Part model, mm, in its own coordinate system. Face numbers are marked on the shaded views. A direction names the side the tool comes from. Round coordinates to 2 decimals unless told otherwise and drop trailing zeros. Loops run counter-clockwise (first coordinate to the right, second up) from the corner with the lowest first, then second, coordinate; pieces in that order, holes last.
(1) Tool access for the marked faces 1 and 2: list every direction of +Z, -Z, +X, -X, +Y, -Y with a clear straight run to the whole face (end or side of a thin tool).
(2) Cut at A-A on x = 0. List the corners of the cut face in (y, z), then the cut area to 3 significant figures.
(3) Cut at D-D on x = -4.5. List the corners of the cut face in (y, z).
(4) Flat gauge pins, fed straight in: pin 1 (1.3 mm diameter, centred on y = -5, z = 2, fed in from +X); pin 2 (6.5 mm diameter, centred on x = 2, z = 10, fed in from -Y); pin 3 (3.5 mm diameter, centred on y = -6, z = 3, fed in from +X). Where does each tip first touch, or does it go through?
(5) Cut at B-B on x = 6.5. List the corners of the cut face in (y, z).
(6) Probe probe 1 along X at (y, z) = (-4.5, 1.2); probe 2 along X at (y, z) = (12.8, 9); probe 3 along Y at (x, z) = (-7, 2). List the from-to ranges inside material, lowest first.
(7) Cut at C-C on y = -4.5. Count the separate pieces of the cut face and the enclosed holes in it, then the cut area to 3 significant figures.
(8) Mould opens along Y. For the marked faces 3, 4, 5 and 6 say: +Y half, -Y half, draft (parallel to the pull), parting line (faces both ways), or undercut.
from build123d import *

# Parameters (mm, degrees)
SKETCH1_W                               = 18
SKETCH1_H                               = 30
BOSS_EXTRUDE1_DEPTH                     = 3
SKETCH3_W                               = 18
SKETCH3_H                               = 3
BOSS_EXTRUDE2_DEPTH                     = 9
CBORE_FOR_M5_HEX_HEAD_BOLT1_D           = 4
CBORE_FOR_M5_HEX_HEAD_BOLT1_DEPTH       = 4
CBORE_FOR_M5_HEX_HEAD_BOLT1_CBORE_D     = 5
CBORE_FOR_M5_HEX_HEAD_BOLT1_CBORE_DEPTH = 0.8
CBORE_FOR_M5_HEX_HEAD_BOLT1_TIP         = 1.178090033
CHAMFER1_SIZE                           = 1
SKETCH8_W                               = 18
SKETCH8_H                               = 6
CUT_EXTRUDE1_DEPTH                      = 12
FILLET2_R                               = 0.5
F_3_0MM_DOWEL_HOLE1_D                   = 3
F_3_0MM_DOWEL_HOLE1_DEPTH               = 10
F_3_0MM_DOWEL_HOLE1_TIP                 = 0.901290929


with BuildPart() as part:
    # Sketch1 → Boss-Extrude1 (new body)
    with BuildSketch(Plane.XY):
        Rectangle(SKETCH1_W, SKETCH1_H)
    extrude(amount=BOSS_EXTRUDE1_DEPTH)

    # Sketch2 → Cut-Revolve1 (revolve, cut)
    with BuildSketch(Plane.XY.offset(3)):
        Polygon((6.8, 8.5), (6, 8.5), (6, 6), (9, 6), (9, 8.5), (8.2, 8.5), (8.2, 8), (6.8, 8), align=None)
    cut_revolve1 = revolve(axis=Axis((6.04728637, 6, 3), (1, 0, 0)), mode=Mode.SUBTRACT)

    # Sketch2<3> → Revolve1 (revolve)
    with BuildSketch(Plane.XY.offset(3), mode=Mode.PRIVATE) as revolve1_sk:
        Polygon((6.8, 9), (6.8, 8.5), (6.8, 8), (8.2, 8), (8.2, 8.5), (9, 8.5), (9, 9), align=None)
    revolve1 = revolve(revolve1_sk.sketch.rotate(Axis((6.04728637, 6, 3), (1, 0, 0)), 90), axis=Axis((6.04728637, 6, 3), (1, 0, 0)))

    # Mirror1: Cut-Revolve1, Revolve1 across plane
    add(cut_revolve1.mirror(Plane(origin=(0, 0, 0), x_dir=(0, 0, 1), z_dir=(1, 0, 0))), mode=Mode.SUBTRACT)
    add(revolve1.mirror(Plane(origin=(0, 0, 0), x_dir=(0, 0, 1), z_dir=(1, 0, 0))))

    # Mirror2: Cut-Revolve1, Revolve1 across plane
    add(cut_revolve1.mirror(Plane.ZX), mode=Mode.SUBTRACT)
    add(revolve1.mirror(Plane.ZX))

    # Mirror2 copy 1 sketch → Mirror2 copy 1 (revolve, cut)
    with BuildSketch(Plane(origin=(0, 0, 3), x_dir=(-1, 0, 0), z_dir=(0, 0, 1))):
        Polygon((6.8, 8.5), (6, 8.5), (6, 6), (9, 6), (9, 8.5), (8.2, 8.5), (8.2, 8), (6.8, 8), align=None)
    revolve(axis=Axis((-6.04728637, -6, 3), (-1, 0, 0)), mode=Mode.SUBTRACT)

    # Mirror2 copy 2 sketch → Mirror2 copy 2 (revolve)
    with BuildSketch(Plane(origin=(0, 0, 3), x_dir=(-1, 0, 0), z_dir=(0, 0, 1))):
        Polygon((6.8, 9), (6.8, 8.5), (6.8, 8), (8.2, 8), (8.2, 8.5), (9, 8.5), (9, 9), align=None)
    revolve(axis=Axis((-6.04728637, -6, 3), (-1, 0, 0)))

    # Sketch3 → Boss-Extrude2 (add)
    with BuildSketch(Plane.XY.offset(3)):
        with Locations((0, 13.5)):
            Rectangle(SKETCH3_W, SKETCH3_H)
    extrude(amount=BOSS_EXTRUDE2_DEPTH)

    # CBORE for M5 Hex Head Bolt1
    with Locations(Plane(origin=(0, 15, 0), x_dir=(1, 0, 0), z_dir=(0, 1, 0))):
        with Locations((-6, -9), (6, -9)):
            CounterBoreHole(CBORE_FOR_M5_HEX_HEAD_BOLT1_D / 2, CBORE_FOR_M5_HEX_HEAD_BOLT1_CBORE_D / 2, CBORE_FOR_M5_HEX_HEAD_BOLT1_CBORE_DEPTH, depth=CBORE_FOR_M5_HEX_HEAD_BOLT1_DEPTH)
            with Locations((0, 0, -(CBORE_FOR_M5_HEX_HEAD_BOLT1_DEPTH + CBORE_FOR_M5_HEX_HEAD_BOLT1_TIP / 2))):  # 119° drill point
                Cone(0, CBORE_FOR_M5_HEX_HEAD_BOLT1_D / 2, CBORE_FOR_M5_HEX_HEAD_BOLT1_TIP, mode=Mode.SUBTRACT)

    # Chamfer1
    chamfer1_edges = [part.edges().sort_by_distance(p)[0] for p in [
        (0, 12, 3),
        (0, 15, 0),
    ]]
    chamfer(chamfer1_edges, length=CHAMFER1_SIZE)

    # Sketch8 → Cut-Extrude1 (cut)
    with BuildSketch(Plane(origin=(0, 0, 0), x_dir=(-1, 0, 0), z_dir=(0, 0, -1))):
        with Locations((0, -12)):
            Rectangle(SKETCH8_W, SKETCH8_H)
    extrude(amount=-CUT_EXTRUDE1_DEPTH, mode=Mode.SUBTRACT)

    # Fillet2
    # the kernel refuses this fillet: 0.5 mm, written as the material it takes off along each edge
    with BuildSketch(Plane(origin=(-10.25, 15, 12), x_dir=(0, 0, -1), z_dir=(1, 0, 0))) as fillet2_piece_1:
        with BuildLine():
            CenterArc((FILLET2_R, -FILLET2_R), FILLET2_R, 90, 90)
            Line((0, -FILLET2_R), (0, 0))
            Line((0, 0), (FILLET2_R, 0))
        make_face()
    extrude(amount=20.5, mode=Mode.SUBTRACT)
    with BuildSketch(Plane(origin=(-9, 6.000000014, 0), x_dir=(1, 0, 0), z_dir=(0, -1, 0))) as fillet2_piece_2:
        with BuildLine():
            CenterArc((FILLET2_R, FILLET2_R), FILLET2_R, 180, 90)
            Line((0, FILLET2_R), (0, 0))
            Line((0, 0), (FILLET2_R, 0))
        make_face()
    extrude(amount=12.000000014, mode=Mode.SUBTRACT)
    with BuildSketch(Plane(origin=(-9, 15.883883476, 1.883883476), x_dir=(0, -0.7071067811865476, 0.7071067811865476), z_dir=(0, -0.7071067811865476, -0.7071067811865476)), Plane(origin=(9, 15.883883476, 1.883883476), x_dir=(-1, 0, 0), z_dir=(0, -0.7071067811865476, -0.7071067811865476))) as fillet2_piece_3:
        with BuildLine():
            CenterArc((FILLET2_R, -FILLET2_R), FILLET2_R, 90, 90)
            Line((0, -FILLET2_R), (0, 0))
            Line((0, 0), (FILLET2_R, 0))
        make_face()
    extrude(amount=3.914213562, mode=Mode.SUBTRACT)
    with BuildSketch(Plane(origin=(9, -6.000000014, 0), x_dir=(-1, 0, 0), z_dir=(0, 1, 0))) as fillet2_piece_4:
        with BuildLine():
            CenterArc((FILLET2_R, FILLET2_R), FILLET2_R, 180, 90)
            Line((0, FILLET2_R), (0, 0))
            Line((0, 0), (FILLET2_R, 0))
        make_face()
    extrude(amount=12.000000015, mode=Mode.SUBTRACT)
    with BuildSketch(Plane(origin=(10.25, -9, 0), x_dir=(0, 0, 1), z_dir=(-1, 0, 0))) as fillet2_piece_5:
        with BuildLine():
            CenterArc((FILLET2_R, FILLET2_R), FILLET2_R, 180, 90)
            Line((0, FILLET2_R), (0, 0))
            Line((0, 0), (FILLET2_R, 0))
        make_face()
    extrude(amount=20.5, mode=Mode.SUBTRACT)
    with BuildSketch(Plane(origin=(9, 15, 13.25), x_dir=(-1, 0, 0), z_dir=(0, 0, -1)), Plane(origin=(-9, 15, -0.25), x_dir=(1, 0, 0), z_dir=(0, 0, 1))) as fillet2_piece_6:
        with BuildLine():
            CenterArc((FILLET2_R, -FILLET2_R), FILLET2_R, 90, 90)
            Line((0, -FILLET2_R), (0, 0))
            Line((0, 0), (FILLET2_R, 0))
        make_face()
    extrude(amount=13.5, mode=Mode.SUBTRACT)
    with BuildSketch(Plane(origin=(9, -10.25, 0), x_dir=(-1, 0, 0), z_dir=(0, 1, 0))) as fillet2_piece_7:
        with BuildLine():
            CenterArc((FILLET2_R, FILLET2_R), FILLET2_R, 180, 90)
            Line((0, FILLET2_R), (0, 0))
            Line((0, 0), (FILLET2_R, 0))
        make_face()
    extrude(amount=4.249999986, mode=Mode.SUBTRACT)
    with BuildSketch(Plane(origin=(9, 6, 0), x_dir=(-1, 0, 0), z_dir=(0, 1, 0))) as fillet2_piece_8:
        with BuildLine():
            CenterArc((FILLET2_R, FILLET2_R), FILLET2_R, 180, 90)
            Line((0, FILLET2_R), (0, 0))
            Line((0, 0), (FILLET2_R, 0))
        make_face()
    extrude(amount=9.25, mode=Mode.SUBTRACT)
    with BuildSketch(Plane(origin=(-9, 15.25, 0), x_dir=(1, 0, 0), z_dir=(0, -1, 0))) as fillet2_piece_9:
        with BuildLine():
            CenterArc((FILLET2_R, FILLET2_R), FILLET2_R, 180, 90)
            Line((0, FILLET2_R), (0, 0))
            Line((0, 0), (FILLET2_R, 0))
        make_face()
    extrude(amount=9.249999986, mode=Mode.SUBTRACT)
    with BuildSketch(Plane(origin=(-9, -6, 0), x_dir=(1, 0, 0), z_dir=(0, -1, 0))) as fillet2_piece_10:
        with BuildLine():
            CenterArc((FILLET2_R, FILLET2_R), FILLET2_R, 180, 90)
            Line((0, FILLET2_R), (0, 0))
            Line((0, 0), (FILLET2_R, 0))
        make_face()
    extrude(amount=4.25, mode=Mode.SUBTRACT)

    # Ø3.0mm Dowel Hole1
    with Locations(Plane(origin=(0, 0, 0), x_dir=(-1, 0, 0), z_dir=(0, 0, -1))):
        with Locations((0, -4.5), (0, 2.8)):
            Hole(F_3_0MM_DOWEL_HOLE1_D / 2, depth=F_3_0MM_DOWEL_HOLE1_DEPTH)
            with Locations((0, 0, -(F_3_0MM_DOWEL_HOLE1_DEPTH + F_3_0MM_DOWEL_HOLE1_TIP / 2))):  # 118° drill point
                Cone(0, F_3_0MM_DOWEL_HOLE1_D / 2, F_3_0MM_DOWEL_HOLE1_TIP, mode=Mode.SUBTRACT)

    # Cut-Extrude2 cone 1 section (through the dimple's axis) → Cut-Extrude2 (revolve, cut)
    with BuildSketch(Plane(origin=(0, 2.8, 3), x_dir=(0, -1, 0), z_dir=(1, 0, 0))):
        Polygon((0, 0), (2.75, 0), (0, 2.75), align=None)
    revolve(axis=Axis((0, 2.8, 3), (0, 0, -1)), mode=Mode.SUBTRACT)

    # Cut-Extrude2 cone 2 section (through the dimple's axis) → Cut-Extrude2 cone 2 (revolve, cut)
    with BuildSketch(Plane(origin=(0, -4.5, 3), x_dir=(0, -1, 0), z_dir=(1, 0, 0))):
        Polygon((0, 0), (2.75, 0), (0, 2.75), align=None)
    revolve(axis=Axis((0, -4.5, 3), (0, 0, -1)), mode=Mode.SUBTRACT)


solid = part.part
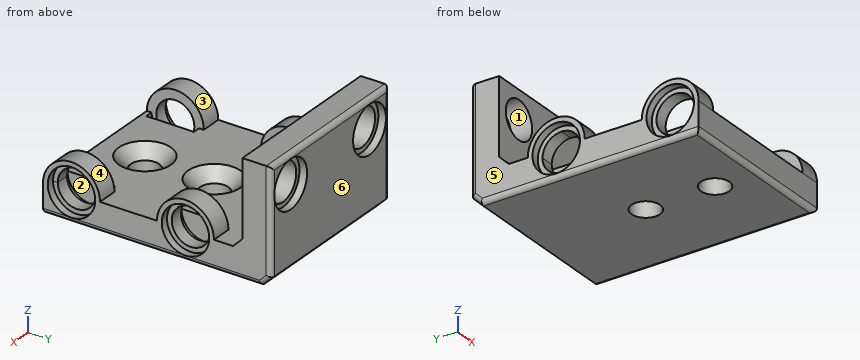
Final values:
1. face 1: +Y, -Y
1. face 2: +Z
2. outline: (-9, 0.5) arc R0.5 ccw to (-8.5, 0) - (-6, 0) - (-6, 1.75) - (-7.25, 3) - (-9, 3) - close; (-3, 0) - (1.3, 0) - (1.3, 1.75) - (0.05, 3) - (-1.75, 3) - (-3, 1.75) - close; (4.3, 0) - (14, 0) - (15, 1) - (15, 11.5) arc R0.5 ccw to (14.5, 12) - (12, 12) - (12, 4) - (11, 3) - (5.55, 3) - (4.3, 1.75) - close
2. area: 77.8 mm2
3. outline: (-9, 0.5) arc R0.5 ccw to (-8.5, 0) - (14, 0) - (15, 1) - (15, 7) - (14.2, 7) - (14.2, 7.68) - (12, 7.68) - (12, 4) - (11, 3) - (-9, 3) - close; (12, 10.32) - (14.2, 10.32) - (14.2, 11) - (15, 11) - (15, 11.5) arc R0.5 ccw to (14.5, 12) - (12, 12) - close
4. pin 1: stops at x = 8.2
4. pin 2: stops at y = 12
4. pin 3: stops at x = 6
5. outline: (-9, 0.5) arc R0.5 ccw to (-8.5, 0) - (14, 0) - (15, 1) - (15, 6.55) - (14.2, 6.55) - (14.2, 7.06) - (12, 7.06) - (12, 4) - (11, 3) - (8.5, 3) arc R2.5 cw to (3.5, 3) - (-3.5, 3) arc R2.5 cw to (-8.5, 3) - (-9, 3) - close; (12, 10.94) - (14.2, 10.94) - (14.2, 11.45) - (15, 11.45) - (15, 11.5) arc R0.5 ccw to (14.5, 12) - (12, 12) - close
6. probe 1: x = -8.2 to -6.8, -6 to -1.5, 1.5 to 6, 6.8 to 8.2
6. probe 2: x = -9 to -8, -4 to 4, 8 to 9
6. probe 3: y = -9 to -7.73, -4.27 to 4.27, 7.73 to 15
7. separate pieces: 4
7. enclosed holes: 0
7. area: 37.8 mm2
8. face 3: undercut
8. face 4: undercut
8. face 5: draft
8. face 6: +Y half
